```python
from build123d import *

# Parameters (mm, degrees)
SKETCH005_AS_DRAWN_W              = 7.5
SKETCH005_AS_DRAWN_H              = 20.5
SKETCH005_AS_DRAWN_H_2            = 16
EXTRUDE_DEPTH                     = 30
EXTRUDE_ONTO_SKETCH005_ROLL_ANGLE = 90
SKETCH_R                          = 20.5
SKETCH003_R                       = 25.5
SKETCH004_R                       = 8.5
POCKET_DEPTH                      = 5
CYLINDER001_R                     = 20.5
CYLINDER001_DEPTH                 = 20
CYLINDER_R                        = 25.5
CYLINDER_DEPTH                    = 20
FILLET_R                          = 3


with BuildPart() as obj1:
    # Sketch005 as drawn → Extrude (new)
    with BuildSketch(Plane.XY):
        with Locations((-8.152101, 32.07517)):
            Rectangle(SKETCH005_AS_DRAWN_W, SKETCH005_AS_DRAWN_H)
        with Locations((9.96979, 29.984642)):
            Rectangle(SKETCH005_AS_DRAWN_W, SKETCH005_AS_DRAWN_H_2)
    extrude(amount=EXTRUDE_DEPTH)


with BuildPart() as obj1_1:
    # Extrude onto Sketch005 roll: moved
    add(obj1.part.rotate(Axis((0, 0, 0), (1, 0, 0)), EXTRUDE_ONTO_SKETCH005_ROLL_ANGLE))


with BuildPart() as obj1_2:
    # Extrude onto Sketch005 placement: moved
    add(obj1_1.part.moved(Location((0, -15, 0))))


with BuildPart() as loft_body:
    # Sketch → Loft section 0
    with BuildSketch(Plane.XY.offset(20)):
        Circle(SKETCH_R)
    # Sketch002 → Loft section 1
    with BuildSketch(Plane.XY.offset(60)):
        with BuildLine():
            Line((-24.999998, 25), (24.999999, 25))
            ThreePointArc((30, 20.000001), (28.540896, 23.540898), (24.999999, 25))
            Line((30, -19.999999), (30, 20.000001))
            ThreePointArc((24.999999, -25), (28.539164, -23.539164), (30, -19.999999))
            Line((-24.999998, -25), (24.999999, -25))
            ThreePointArc((-30, -19.999999), (-28.527665, -23.527666), (-24.999998, -25))
            Line((-30, 19.999997), (-30, -19.999999))
            ThreePointArc((-24.999998, 25), (-28.522614, 23.522614), (-30, 19.999997))
        make_face()
    loft()


with BuildPart() as pocket:
    # Sketch003 → Loft001 section 0
    with BuildSketch(Plane.XY.offset(20)):
        Circle(SKETCH003_R)
    # Sketch001 → Loft001 section 1
    with BuildSketch(Plane.XY.offset(65)):
        with BuildLine():
            Line((-35, -24.999999), (-35, 25))
            ThreePointArc((-30, 30), (-33.52786, 28.52786), (-35, 25))
            Line((-30, 30), (29.999999, 30))
            ThreePointArc((35, 25), (33.544012, 28.544013), (29.999999, 30))
            Line((35, 25), (35, -25.000001))
            ThreePointArc((30.000001, -30), (33.536169, -28.536168), (35, -25.000001))
            Line((-30.000003, -30), (30.000001, -30))
            ThreePointArc((-35, -24.999999), (-33.539778, -28.539776), (-30.000003, -30))
        make_face()
    loft()

    # Cut001: cut Loft body
    add(loft_body.part, mode=Mode.SUBTRACT)

    # Sketch004 → Pocket (cut)
    with BuildSketch(Plane.XY.offset(65)):
        with Locations((-13, 0)):
            Circle(SKETCH004_R)
        with Locations((13, 0)):
            Circle(SKETCH004_R)
    extrude(amount=-POCKET_DEPTH, mode=Mode.SUBTRACT)


with BuildPart() as cut002:
    # Sketch006 → Loft002 section 0
    with BuildSketch(Plane.XY.offset(20)):
        Polygon((20, -15), (20, -26.992193), (-20, -26.992193), (-20, -15), (0, -25), align=None)
    # Sketch007 → Loft002 section 1
    with BuildSketch(Plane.XY.offset(65)):
        Polygon((-20, -30), (20, -30), (20, -26.285252), (0, -28.799719), (-20, -26.499249), align=None)
    loft()

    # Fusion: union Pocket
    add(pocket.part)

    # Cut002: cut obj1
    add(obj1_2.part, mode=Mode.SUBTRACT)


with BuildPart() as obj2:
    # Cylinder001 → Cylinder001 (new body)
    with BuildSketch(Plane.XY):
        Circle(CYLINDER001_R)
    extrude(amount=CYLINDER001_DEPTH)


with BuildPart() as fusion001:
    # Cylinder → Cylinder (new body)
    with BuildSketch(Plane.XY):
        Circle(CYLINDER_R)
    extrude(amount=CYLINDER_DEPTH)

    # Cut: cut obj2
    add(obj2.part, mode=Mode.SUBTRACT)

    # Fillet
    fillet_edges = [fusion001.edges().sort_by_distance(p)[0] for p in [
        (-25.5, 0, 0),
    ]]
    fillet(fillet_edges, radius=FILLET_R)

    # Fusion001: union Cut002
    add(cut002.part)


solid = fusion001.part
```
Could you check a few things on this model? Use its own coordinates, in mm. A direction names the side the tool comes from. Round coordinates to 2 decimals unless told otherwise and drop trailing zeros. Loops run counter-clockwise (first coordinate to the right, second up) from the corner with the lowest first, then second, coordinate; pieces in that order, holes last. Notation, with made-up numbers: M 86.25,-27 L 122.25,-27 A28 cw 122.25,10 Z; hole C 19.25,9 d6. An arc over 180 degrees is marked long. Answer as CSV lines item,"result".
1) Imagine slicing it at B-B on x = -8. Count the separate pieces of the cut face and the enclosed holes in it, and give its area (3 significant figures).
From the geometry:
separate pieces,"3"
enclosed holes,"0"
area,"738 mm^2"
2) Which directions (+Z, -Z, +X, -X, +Y, -Y) give clear straight access to the entire face, cutting with the end or side of a thin tool? Please do faces 4 (the cylindrical face through (4.51, 0.37, 62.54)), 5 (the cylindrical face through (-4.444, -20.013, 9.86)), 6 (the flat face through (0, 0, 60)), 7 (the flat face through (-11.902, -24, 32)).
From the geometry:
face 4,"+Z"
face 5,"-Z"
face 6,"none"
face 7,"-Y"
3) For pin 1 Ø10 at (x, z) = (10, 48.5) entering from -Y; pin 2 Ø3 at (x, z) = (-23.5, 19) entering from +Y; pin 3 Ø9 at (y, z) = (-22, 27.5) entering from +X, each with a flat end and sliding along its axis, tell me the tip position at first contact or that it passes through.
From the geometry:
pin 1,"y = -29.23"
pin 2,"y = 12.89"
pin 3,"x = 23.29"
4) If I drill on probe 1 along Y at (x, z) = (0, 14); probe 2 along Y at (x, z) = (13, 61), over which ranges is the centre line in solid material (lowest first)?
From the geometry:
probe 1,"-25.5 to -20.5, 20.5 to 25.5"
probe 2,"-29.73 to -8.5, 8.5 to 29.46"
5) We'd pull the mould along X, two halves only. Please class faces 1 (the flat face through (9.9, -18.2, 0)), 2 (the flat face through (-4.402, -24, 32)), 3 (the cylindrical face through (-5.5, -24.9, 11.4)): released by +X, released by -X, zero draft, split by the parting line, or undercut.
From the geometry:
face 1,"zero draft"
face 2,"undercut"
face 3,"split by the parting line"
6) Imagine slicing it at A-A on z = 8.5. List the corners of the cut face in (x, y) for me.
From the geometry:
outline,"C 0,0 d51; hole C 0,0 d41"
